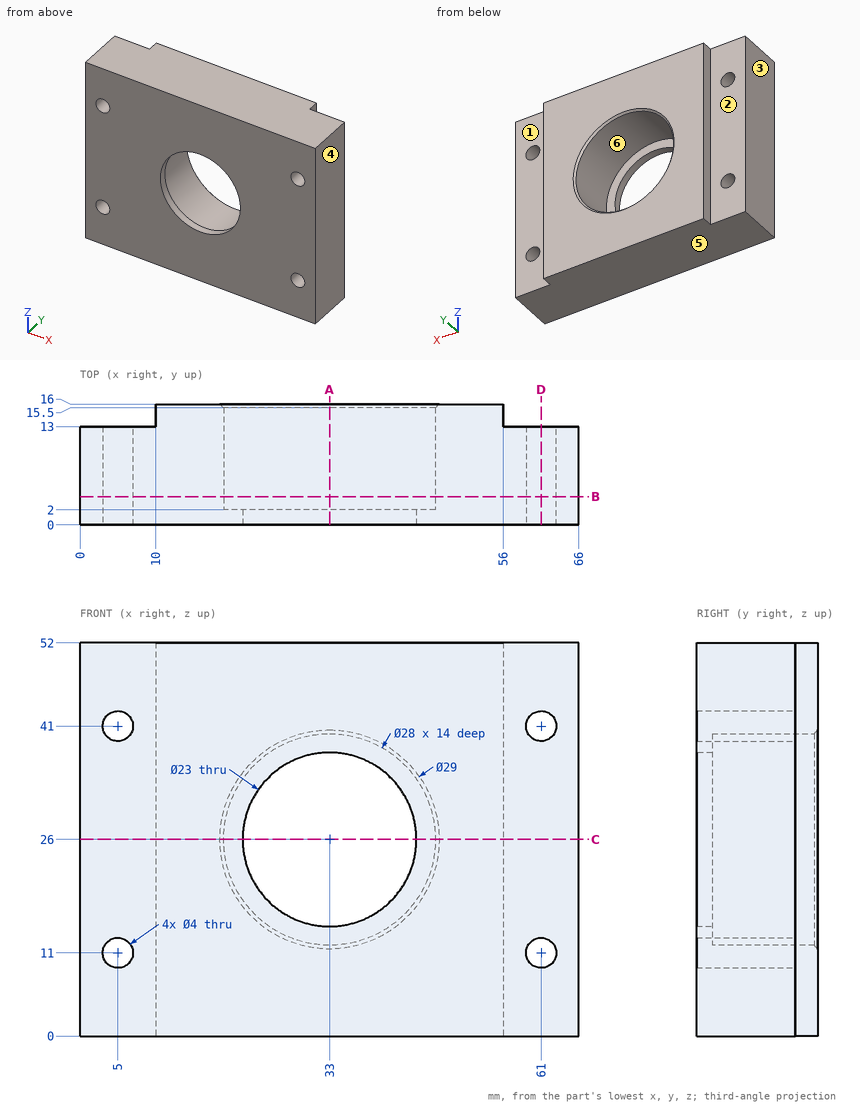
Design review of the part shown in the three views and the two pictorial views. Dimensions are in mm from the part's minimum x, y and z. A direction names the side the tool comes from. Round coordinates to 2 decimals unless told otherwise and drop trailing zeros. Write each loop counter-clockwise with the first axis right and the second up, starting at its lowest first coordinate (ties: lowest second). Pieces come first, ordered by that corner, then holes. Notation, with made-up numbers: (-10, 79) -> (16, 79) arc R21 cw to (16, 85) -> close; hole circle Ø6 at (-22, 15.5). An arc over 180 degrees is marked (long way). One line per question, with ' | ' between items. Start each with the question number.
1) For pin 1 Ø5 at (x, z) = (5, 11) entering from -Y; pin 2 Ø8 at (x, z) = (2.5, 39) entering from +Y; pin 3 Ø0.9 at (y, z) = (14.5, 18.5) entering from +X; pin 4 Ø1.5 at (y, z) = (14, 20) entering from -X, all flat-tipped, find the tip position at first contact; note any pin that passes through.
2) Add section D-D (x = 61). Write out the cut boundary in (y, z), and give its area (3 significant figures).
3) Add section A-A (x = 33). Write out the cut boundary in (y, z).
4) Machinability: for the marked faces 1, 2 and 3, which of the approach directions +Z, -Z, +X, -X, +Y, -Y give a long, thin tool a straight path to every point of the face, cutting with its end or side? Answer none if there is none.
5) Add section B-B (y = 3.75). Write out the cut boundary in (x, z), and give its area (3 significant figures).
6) Add section C-C (z = 26). Write out the cut boundary in (x, y).
7) Wall thickness on line 1 along Z through (x, y) = (61, 5.25); line 2 along Z through (x, y) = (6.5, 12.75); line 3 along X through (y, z) = (6.5, 34): over which ranges is each line inside the solid? List them lowest first.
8) Mouldability with a two-part tool opening along X and no side actions: class the marked faces 4, 5 and 6 as +X half, -X half, draft (parallel to the pull), parting line (faces both ways), or undercut.
Reported:
1) pin 1: stops at y = 0 | pin 2: stops at y = 13 | pin 3: stops at x = 56 | pin 4: stops at x = 10
2) outline: (0, 0) -> (13, 0) -> (13, 9) -> (0, 9) -> close; (0, 13) -> (13, 13) -> (13, 39) -> (0, 39) -> close; (0, 43) -> (13, 43) -> (13, 52) -> (0, 52) -> close | area: 572 mm²
3) outline: (0, 0) -> (16, 0) -> (16, 11.5) -> (15.5, 12) -> (2, 12) -> (2, 14.5) -> (0, 14.5) -> close; (0, 37.5) -> (2, 37.5) -> (2, 40) -> (15.5, 40) -> (16, 40.5) -> (16, 52) -> (0, 52) -> close
4) face 1: +Z, -Z, +X, +Y | face 2: +Z, -Z, -X, +Y | face 3: +Z, -Z, -X, +Y, -Y
5) outline: (0, 0) -> (66, 0) -> (66, 52) -> (0, 52) -> close; hole circle Ø4 at (5, 11); hole circle Ø4 at (5, 41); hole circle Ø28 at (33, 26); hole circle Ø4 at (61, 11); hole circle Ø4 at (61, 41) | area: 2,770 mm²
6) outline: (0, 0) -> (21.5, 0) -> (21.5, 2) -> (19, 2) -> (19, 15.5) -> (18.5, 16) -> (10, 16) -> (10, 13) -> (0, 13) -> close; (44.5, 0) -> (66, 0) -> (66, 13) -> (56, 13) -> (56, 16) -> (47.5, 16) -> (47, 15.5) -> (47, 2) -> (44.5, 2) -> close
7) line 1: z = 0 to 9, 13 to 39, 43 to 52 | line 2: z = 0 to 9.68, 12.32 to 39.68, 42.32 to 52 | line 3: x = 0 to 21.51, 44.49 to 66
8) face 4: +X half | face 5: draft | face 6: undercut
